Could you check a few things on this model? Use its own coordinates, in mm. A direction names the side the tool comes from. Round coordinates to 2 decimals unless told otherwise and drop trailing zeros. Write each loop counter-clockwise with the first axis right and the second up, starting at its lowest first coordinate (ties: lowest second). Pieces come first, ordered by that corner, then holes. Notation, with made-up numbers: (-21, 55.25) - (21, 55.25) arc R17 ccw to (21, 88.25) - close; hole circle Ø5 at (59, 53.5). An arc over 180 degrees is marked (long way). Put each result on its own line as item: value.
from build123d import *

# Parameters (mm, degrees)
F0_W          = 46
F0_H          = 3
F1_DEPTH      = 22
F2_R          = 5
F2_R_2        = 2
F3_DEPTH      = 22.001
F3_DEPTH_BACK = 22.001
F4_DEPTH      = 12
F5_W          = 5
F5_H          = 5
F6_DEPTH      = 5
F8_DEPTH      = 5.001


with BuildPart() as f1:
    # F0 (on Front) → F1 (new body, symmetric)
    with BuildSketch(Plane.XZ):
        Rectangle(F0_W, F0_H)
    extrude(amount=F1_DEPTH, both=True)

    # F2 (on Front) → F3 (cut, two sides)
    with BuildSketch(Plane.XZ) as f3_sk:
        with Locations((-23, -3.5)):
            Circle(F2_R)
        with Locations((-23, -3.5)):
            Circle(F2_R_2, mode=Mode.SUBTRACT)
    extrude(amount=F3_DEPTH, mode=Mode.SUBTRACT)
    extrude(f3_sk.sketch, amount=-F3_DEPTH_BACK, mode=Mode.SUBTRACT)

    # F2 (on Front) → F4 (join, symmetric)
    with BuildSketch(Plane.XZ):
        with Locations((-23, -3.5)):
            Circle(F2_R)
        with Locations((-23, -3.5)):
            Circle(F2_R_2, mode=Mode.SUBTRACT)
    extrude(amount=F4_DEPTH, both=True)

    # F5 (on face) → F6 (join)
    with BuildSketch(Plane(origin=(0, 0, -1.5), x_dir=(1, 0, 0), z_dir=(0, 0, -1))):
        with Locations((20.5, 19.5)):
            Rectangle(F5_W, F5_H)
    extrude(amount=F6_DEPTH)

    # F7 (on face) → F8 (cut, through all)
    with BuildSketch(Plane(origin=(0, -17, 0), x_dir=(-1, 0, 0), z_dir=(0, 1, 0))):
        Polygon((-23, -1.5), (-23, -6.5), (-20, -6.5), (-21.5, -1.5), align=None)
    extrude(amount=-F8_DEPTH, mode=Mode.SUBTRACT)


solid = f1.part
(1) Imagine slicing it at C-C, the plane x = -13. List the corners of the cut face in (y, z) for me.
Values found:
outline: (-22, -1.5) - (22, -1.5) - (22, 1.5) - (-22, 1.5) - close
(2) Imagine slicing it at B-B, the plane y = 7.5. List the corners of the cut face in (x, z) for me.
Values found:
outline: (-23, 1.5) arc R5 ccw (long way) to (-18.42, -1.5) - (23, -1.5) - (23, 1.5) - close; hole circle Ø4 at (-23, -3.5)
(3) Imagine slicing it at A-A, the plane z = -3.5. List the corners of the cut face in (x, y) for me, then the cut area to 4 significant figures.
Values found:
outline: (-28, -12) - (-25, -12) - (-25, 12) - (-28, 12) - close; (-21, -12) - (-18, -12) - (-18, 12) - (-21, 12) - close; (18, -22) - (20.9, -22) - (20.9, -17) - (18, -17) - close
area: 158.5 mm^2
(4) I'm going to push flat-ended pins straight in: pin 1 (5 mm diameter, centred on x = -24, z = -3.5, fed in from +Y); pin 2 (5 mm diameter, centred on x = -2, y = 9.5, fed in from -Z); pin 3 (3 mm diameter, centred on x = 16.5, z = -2.5, fed in from +Y); pin 4 (3 mm diameter, centred on x = -22.5, z = -3, fed in from -Y). Where does each tip first touch, or does it pass through?
Values found:
pin 1: stops at y = 12
pin 2: stops at z = -1.5
pin 3: stops at y = 22
pin 4: stops at y = -12
(5) Please list where these lines run through material, in increasing order: probe 1 along X at (y, z) = (-2, -4); probe 2 along Y at (x, z) = (-20.5, -7); probe 3 along X at (y, z) = (-6.5, -3.75). Write a range as from..to.
Values found:
probe 1: x = -27.97..-24.94, -21.06..-18.03
probe 2: y = -12..12
probe 3: x = -27.99..-24.98, -21.02..-18.01
(6) If we mould it in two halves opening along X, with no side actions, what happens to faces 6 (the face through (-25.89, -0.17, -7.58)), 7 (the face through (2, 0, -1.5)), 8 (the face through (-24.6, 0.2, -4.7))? For each: pulls with the +X half, pulls with the -X half, needs draft (parallel to the pull), parting line crosses it, or undercut.
Values found:
face 6: parting line crosses it
face 7: needs draft
face 8: undercut
(7) Imagine slicing it at D-D, the plane y = 18.5. List the corners of the cut face in (x, z) for me, then the cut area to 3 significant figures.
Values found:
outline: (-23, 1.5) arc R5 cw to (-18.42, -1.5) - (23, -1.5) - (23, 1.5) - close
area: 128 mm^2
(8) For faces 1 (the face through (18, -19, -4)), 2 (the face through (-23, -12, -6)), 3 (the face through (-20.228, 17.07, 0.661)), 4 (the face through (19, -17, -4)), 5 (the face through (19, -20, -6.5)), which set-ups out of +Z, -Z, +X, -X, +Y, -Y let a thin tool reach every point of the face, with its end or its side?
Values found:
face 1: -Z, -X, +Y, -Y
face 2: -Z, -X, -Y
face 3: -Z, -X, +Y
face 4: -Z, +X, -X, +Y
face 5: -Z, +X, -X, +Y, -Y
